Source: three-view drawing plus pictorial views. Frame: mm from the lowest corner of the part. A direction names the side the tool comes from. Give positions to 0.01 mm unless a question says otherwise; leave off trailing zeros. Loops run counter-clockwise (first coordinate to the right, second up) from the corner with the lowest first, then second, coordinate; pieces in that order, holes last. Notation, with made-up numbers: (-35.5, -18.5) -> (15.5, -18.5) arc R30 cw to (15.5, 4.5) -> close; hole circle Ø4 at (-18, 1). An arc over 180 degrees is marked (long way). Put each result on its own line as item: value.
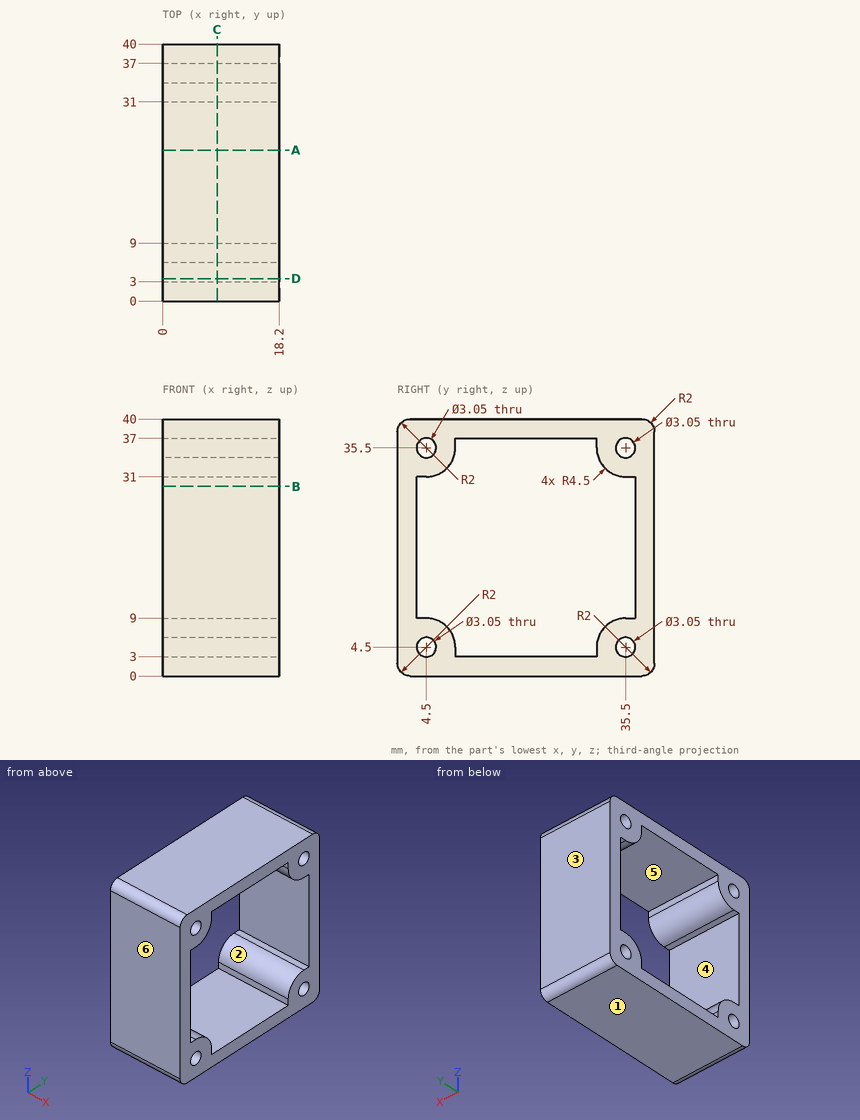
(1) Reachability of the marked faces 5 and 6 from +Z, -Z, +X, -X, +Y, -Y: full face, straight path, thin tool, end or side. Return the list, or none.
Calculated:
face 5: +X, -X
face 6: +Z, -Z, +X, -X, -Y
(2) Line query: probe 1 along Y at (x, z) = (13, 4.5) (3 decimals); probe 2 along Z at (x, y) = (16.75, 12); probe 3 along Z at (x, y) = (8.75, 35). Output: solid intervals per line, ascending. Write a range as from..to.
Calculated:
probe 1: y = 0..2.975, 6.025..9, 31..33.975, 37.025..40
probe 2: z = 0..3, 37..40
probe 3: z = 0..3.06, 5.94..8.97, 31.03..34.06, 36.94..40
(3) Section D-D on y = 3.5. Return loops of the section in (x, z).
Calculated:
outline: (0, 0) -> (18.2, 0) -> (18.2, 3.35) -> (0, 3.35) -> close; (0, 5.65) -> (18.2, 5.65) -> (18.2, 9) -> (0, 9) -> close; (0, 31) -> (18.2, 31) -> (18.2, 34.35) -> (0, 34.35) -> close; (0, 36.65) -> (18.2, 36.65) -> (18.2, 40) -> (0, 40) -> close
(4) Draft query along Z for the marked faces 1, 2, 3 and 4. Return one class per face: released by +Z, released by -Z, zero draft, split by the parting line, or undercut.
Calculated:
face 1: released by -Z
face 2: undercut
face 3: zero draft
face 4: undercut
(5) First-contact query: P1, Ø2.5, axis at y = 35.5, z = 4.5, coming from the -X side. Flat tip, straight axial feed; report the tip coordinate or a pass-through.
Calculated:
P1: passes through
(6) Section C-C on x = 8.5. Return loops of the section in (y, z) (3 decimals).
Calculated:
outline: (0, 2) arc R2 ccw to (2, 0) -> (38, 0) arc R2 ccw to (40, 2) -> (40, 38) arc R2 ccw to (38, 40) -> (2, 40) arc R2 ccw to (0, 38) -> close; hole circle Ø3.05 at (4.5, 4.5); hole circle Ø3.05 at (4.5, 35.5); hole (3, 9) -> (4.5, 9) arc R4.5 cw to (9, 4.5) -> (9, 3) -> (31, 3) -> (31, 4.5) arc R4.5 cw to (35.5, 9) -> (37, 9) -> (37, 31) -> (35.5, 31) arc R4.5 cw to (31, 35.5) -> (31, 37) -> (9, 37) -> (9, 35.5) arc R4.5 cw to (4.5, 31) -> (3, 31) -> close; hole circle Ø3.05 at (35.5, 4.5); hole circle Ø3.05 at (35.5, 35.5)
(7) Section A-A on y = 23.5. Return loops of the section in (x, z).
Calculated:
outline: (0, 0) -> (18.2, 0) -> (18.2, 3) -> (0, 3) -> close; (0, 37) -> (18.2, 37) -> (18.2, 40) -> (0, 40) -> close
